Autodesk Fusion 360 part; units mm, degrees
sketch "Sketch1" plane through (0, 0, 0) normal (0, 0, 1) x (1, 0, 0)
  line L0 (0, 0) -> (15, 0)
  line L1 (15, 0) -> (15, 20)
  line L2 (15, 20) -> (0, 20)
  line L3 (0, 20) -> (0, 0)
  dimension "d1" = 15
  dimension "d2" = 20
extrude "Extrude1" add sketch "Sketch1" along normal blind 1.3
sketch "Sketch3" plane through (0, 0, 1.3) normal (0, 0, 1) x (-1, 0, 0)
  line L0 (0, -20) -> (0, 0)
  line L1 (0, 0) -> (-15, 0)
  line L2 (-15, 0) -> (-15, -20)
  line L3 (-15, -20) -> (0, -20)
  line L4 (-8.65, -4.5) -> (-8.65, -20)
  line L5 (-8.65, -20) -> (-7.5, -20)
  line L6 (-6.35, -4.5) -> (-6.35, -20)
  line L7 (-6.35, -20) -> (-7.5, -20)
  line L8 (-6.35, -3) -> (-8.65, -3)
  line L9 (-6.35, -4.5) -> (-6.35, -3)
  line L10 (-8.65, -4.5) -> (-8.65, -3)
  dimension "d14" = 3
extrude "Extrude2" cut sketch "Sketch3" against normal blind 6 contours L3 L4 L5 L6 L7 L8 L9 L10
sketch "Sketch4" plane through (0, 0, 1.3) normal (0, 0, 1) x (-1, 0, 0)
  line L0 (-6.35, -3) -> (-6.35, -20)
  line L1 (-6.35, -20) -> (0, -20)
  line L2 (0, -20) -> (0, 0)
  line L3 (0, 0) -> (-15, 0)
  line L4 (-15, 0) -> (-15, -20)
  line L5 (-15, -20) -> (-8.65, -20)
  line L6 (-8.65, -20) -> (-8.65, -3)
  line L7 (-8.65, -3) -> (-6.35, -3)
  line L8 (0, 0) -> (-15, 0)
  line L9 (-15, 0) -> (-15, -20)
  line L10 (-15, -20) -> (0, -20)
  line L11 (0, -20) -> (0, 0)
extrude "Extrude3" add sketch "Sketch4" along normal blind 30
sketch "Sketch5" plane through (0, 0, 0) normal (-1, 0, 0) x (0, -1, 0)
  line L0 (-20, 0) -> (0, 0)
  line L1 (0, 0) -> (0, 31.3)
  line L2 (0, 31.3) -> (-20, 31.3)
  line L3 (-20, 31.3) -> (-20, 0)
  line L4 (-10, 31.3) -> (-17, 31.3)
  line L5 (-10, 31.3) -> (-3, 31.3)
  line L6 (-17, 31.3) -> (-17, 23.8)
  line L7 (-3, 31.3) -> (-3, 23.8)
  line L8 (-17, 23.8) -> (-3, 23.8)
  dimension "d19" = 7
  dimension "d20" = 7
  dimension "d21" = 7.5
  dimension "d22" = 7.5
extrude "Extrude4" cut sketch "Sketch5" against normal blind 24 contours L2 L4 L5 L6 L7 L8
sketch "Sketch6" plane through (0, 20, 0) normal (0, 1, 0) x (-1, 0, 0)
  line L0 (-6.35, 1.3) -> (-6.35, 0)
  line L1 (-6.35, 0) -> (0, 0)
  line L2 (0, 0) -> (0, 31.3)
  line L3 (0, 31.3) -> (-15, 31.3)
  line L4 (-15, 31.3) -> (-15, 0)
  line L5 (-15, 0) -> (-8.65, 0)
  line L6 (-8.65, 0) -> (-8.65, 1.3)
  line L7 (-8.65, 1.3) -> (-6.35, 1.3)
  circle A0 centre (-7.5, 27.8) radius 2
  dimension "d26" = 4
extrude "Extrude5" cut sketch "Sketch6" against normal blind 22 contours A0
Source: CAD feature listing. Evaluate the final solid. Frame: model axes, mm. A direction names the side the tool comes from. Give positions to 0.01 mm unless a question says otherwise; leave off trailing zeros. Loops run counter-clockwise (first coordinate to the right, second up) from the corner with the lowest first, then second, coordinate; pieces in that order, holes last. Notation, with made-up numbers: (59, 11) - (84, 11) arc R11 cw to (84, 26) - close; hole circle Ø3 at (43.25, -34). An arc over 180 degrees is marked (long way). Use CSV: the item, a comma, the result in double quotes.
1) Cut plane D-D (x = 11.25). Output: boundary loops of the cut face in (y, z), and give its area (3 significant figures).
Worked out:
outline,"(0, 0) - (20, 0) - (20, 31.3) - (17, 31.3) - (17, 23.8) - (3, 23.8) - (3, 31.3) - (0, 31.3) - close"
area,"521 mm^2"
2) Cut plane A-A (x = 7.5). Output: boundary loops of the cut face in (y, z), and give its area (3 significant figures).
Worked out:
outline,"(0, 0) - (3, 0) - (3, 1.3) - (20, 1.3) - (20, 25.8) - (17, 25.8) - (17, 23.8) - (3, 23.8) - (3, 25.8) - (0, 25.8) - close; (0, 29.8) - (3, 29.8) - (3, 31.3) - (0, 31.3) - close; (17, 29.8) - (20, 29.8) - (20, 31.3) - (17, 31.3) - close"
area,"475 mm^2"
3) Mould query, pull axis X, two halves, no side actions, for faces 1 (the flat face through (8, 20, 15)), 2 (the flat face through (8, 11, 1.3)), 3 (the cylindrical face through (7.76, 1.521, 29.783)), 4 (the flat face through (0, 10, 12)). Classes: +X half, -X half, draft (parallel to the pull), parting line (faces both ways), or undercut.
Worked out:
face 1,"draft"
face 2,"undercut"
face 3,"undercut"
face 4,"-X half"
4) Cut plane C-C (y = 18.5). Output: boundary loops of the cut face in (x, z), and give its area (3 significant figures).
Worked out:
outline,"(0, 0) - (6.35, 0) - (6.35, 1.3) - (8.65, 1.3) - (8.65, 0) - (15, 0) - (15, 31.3) - (0, 31.3) - close; hole circle Ø4 at (7.5, 27.8)"
area,"454 mm^2"
5) Cut plane B-B (z = 27.8). Output: boundary loops of the cut face in (x, y).
Worked out:
outline,"(0, 0) - (5.5, 0) - (5.5, 3) - (0, 3) - close; (0, 17) - (5.5, 17) - (5.5, 20) - (0, 20) - close; (9.5, 0) - (15, 0) - (15, 3) - (9.5, 3) - close; (9.5, 17) - (15, 17) - (15, 20) - (9.5, 20) - close"
6) Pin query (flat end, axial travel): P1, Ø0.6, axis at x = 7.5, z = 0.5, coming from the +Y side; P2, Ø3.5, axis at x = 7.5, z = 27.8, coming from the -Y side. Return the tip coordinate at first contact, or that it passes through.
Worked out:
P1,"stops at y = 3"
P2,"passes through"
7) Set-up query: faces 5 (the flat face through (6.35, 11, 1)), 6 (the cylindrical face through (7.76, 18.521, 29.783)), 7 (the flat face through (6, 17, 26)). Return all of +Z, -Z, +X, -X, +Y, -Y with unobstructed straight access to the full face (end or side cutting, diameter ignored); none if empty.
Worked out:
face 5,"-Z, +Y"
face 6,"+Y, -Y"
face 7,"+Z, +X, -X"
8) Line query: line 1 (Y direction, x = 7, z = 24); line 2 (Z direction, x = 7.5, y = 17.7); line 3 (Z direction, x = 7.5, y = 0.6). Output: solid intervals per line, ascending.
Worked out:
line 1,"y = 0 to 3, 17 to 20"
line 2,"z = 1.3 to 25.8, 29.8 to 31.3"
line 3,"z = 0 to 25.8, 29.8 to 31.3"
